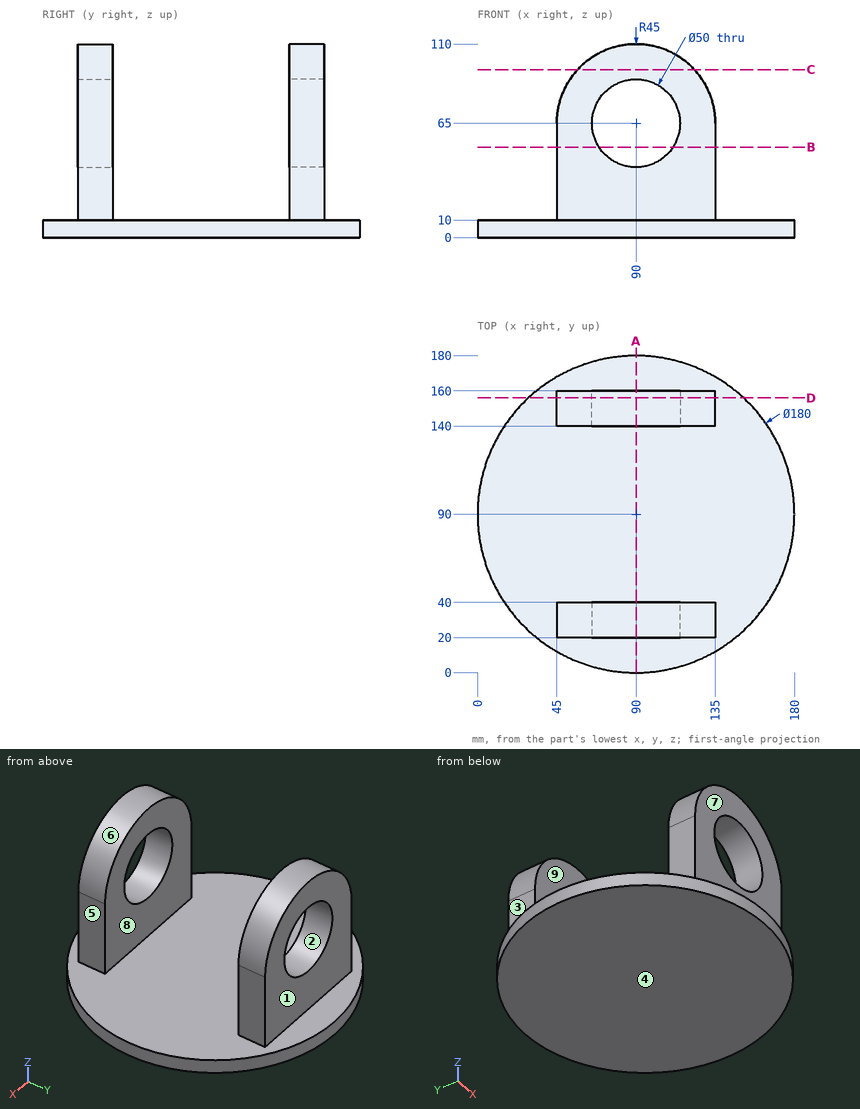
Verification items for this drawing (mm, ordinates from the low corner). A direction names the side the tool comes from. Round coordinates to 2 decimals unless told otherwise and drop trailing zeros. Loops run counter-clockwise (first coordinate to the right, second up) from the corner with the lowest first, then second, coordinate; pieces in that order, holes last. Notation, with made-up numbers: (20.25, 10.25) - (72.25, 10.25) arc R9 ccw to (72.25, 14.25) - close; hole circle Ø7 at (65.25, -35.75). An arc over 180 degrees is marked (long way). Write item = value, one per line.
Q1. Sectioned sample at A-A on x = 90. Record the boundary of the cut face in (y, z), plus the area to 3 significant figures.
Here are the results:
outline = (0, 0) - (180, 0) - (180, 10) - (160, 10) - (160, 40) - (140, 40) - (140, 10) - (40, 10) - (40, 40) - (20, 40) - (20, 10) - (0, 10) - close; (20, 90) - (40, 90) - (40, 110) - (20, 110) - close; (140, 90) - (160, 90) - (160, 110) - (140, 110) - close
area = 3,800 mm^2
Q2. Sectioned sample at B-B on z = 51.5. Record the boundary of the cut face in (x, y).
Here are the results:
outline = (45, 20) - (68.96, 20) - (68.96, 40) - (45, 40) - close; (45, 140) - (68.96, 140) - (68.96, 160) - (45, 160) - close; (111.04, 20) - (135, 20) - (135, 40) - (111.04, 40) - close; (111.04, 140) - (135, 140) - (135, 160) - (111.04, 160) - close
Q3. Depth check by flat-ended pin: pin 1 (10 mm diameter, centred on y = 37.5, z = 26, fed in from +X); pin 2 (3 mm diameter, centred on x = 112, z = 50, fed in from +Y); pin 3 (8 mm diameter, centred on x = 133.5, z = 53.5, fed in from -Y). Enter the tip coordinate at first touch or a pass-through.
Here are the results:
pin_1 = 135
pin_2 = 160
pin_3 = 20
Q4. Material ranges on L1, parallel to Z at x = 90, y = 29.5; L2, parallel to Y at x = 72, z = 43.5; L3, parallel to Z at x = 11.5, y = 131.5, recorded low to high.
Here are the results:
L1 = 0 to 40, 90 to 110
L2 = 20 to 40, 140 to 160
L3 = 0 to 10
Q5. Sectioned sample at C-C on z = 95.5. Record the boundary of the cut face in (x, y).
Here are the results:
outline = (56.91, 20) - (123.09, 20) - (123.09, 40) - (56.91, 40) - close; (56.91, 140) - (123.09, 140) - (123.09, 160) - (56.91, 160) - close
Q6. Sectioned sample at D-D on y = 156. Record the boundary of the cut face in (x, z), plus the area to 3 significant figures.
Here are the results:
outline = (28.81, 0) - (151.19, 0) - (151.19, 10) - (135, 10) - (135, 65) arc R45 ccw to (45, 65) - (45, 10) - (28.81, 10) - close; hole circle Ø50 at (90, 65)
area = 7,390 mm^2
Q7. Tool access check on the marked faces 1, 2, 3, 4 and 5. Record the directions out of +Z, -Z, +X, -X, +Y, -Y that give a thin tool (end or side, any length) a straight path to the whole face; none if there is none.
Here are the results:
face_1 = +Z, +X, -X, +Y
face_2 = +Y, -Y
face_3 = +Z, -X, +Y, -Y
face_4 = -Z, +X, -X, +Y, -Y
face_5 = +Z, +X, +Y, -Y
Q8. Mould release check, pull along Y, two halves, no side actions. Record for the marked faces 6, 7, 8 and 9: +Y half, -Y half, draft (parallel to the pull), parting line (faces both ways), or undercut.
Here are the results:
face_6 = draft
face_7 = -Y half
face_8 = undercut
face_9 = undercut
